Read the model definition and answer for the solid it produces. Units are mm, in the model's axes. A direction names the side the tool comes from. Coordinates: 2 decimals unless noted, no trailing zeros. Order: outer loops, then holes, each group sorted by start corner. A loop starts at its lowest first (then second) coordinate and runs counter-clockwise, first axis right, second up. Notation, with made-up numbers: (43, 20) -> (94, 20) arc R37 ccw to (94, 57) -> close; hole circle Ø2 at (-1.75, -36.75). An arc over 180 degrees is marked (long way). Answer as a JSON object with one key per item and string values. Group by question number.
1) A tool of negligible diameter and unlimited length cuts with its end or side. For faces 1 (the flat face through (-6, -19.05, 19)), 2 (the flat face through (0, -24, 22)), 3 (the flat face through (-6, -28, 25.4)), from which of +Z, -Z, +X, -X, +Y, -Y can it reach the whole face along a straight path? Write none if from no direction.
2) Section B-B on y = -25.5 is taken. Determine the outline of the cut face in (x, z), and give its area (3 significant figures).
3) Consider L1, parallel to Y at x = -6.5, z = 23; L2, parallel to X at y = -3, z = 9.5; L3, parallel to Z at x = -1, y = -9.5. Determine where each line is inside the solid, lowest interval first.
4) Given pin 1 (8 mm diameter, centred on x = -8, z = 18.5, fed in from +Y); pin 2 (6 mm diameter, centred on x = 3.5, y = -4.5, fed in from +Z); pin 3 (12 mm diameter, centred on x = 9.5, y = -27.5, fed in from +Z), each flat-ended and moving along its own axis, determine where each tip first touches the part or whether it passes through.
5) Section A-A on x = -6 is taken. Determine the outline of the cut face in (y, z), and give its area (3 significant figures).
from build123d import *

# Parameters (mm, degrees)
F0_W     = 38.1
F0_H     = 25.4
F1_DEPTH = 12.7
F2_SIZE2 = 25.39999
F2_SIZE  = 38.09999
F4_DEPTH = 12.7


# Not quite as in the source:
# - a fillet or chamfer is up to 0.001 mm smaller than in the source, because OpenCascade refuses the exact size


with BuildPart() as f1:
    # F0 (on Right) → F1 (new body)
    with BuildSketch(Plane.YZ):
        with Locations((-19.05, 12.7)):
            Rectangle(F0_W, F0_H)
    extrude(amount=F1_DEPTH)

    # F2 (size 38.1 and 25.4 in the source; OpenCascade refuses exactly that, so slightly less here)
    f2_edges = [f1.edges().sort_by_distance(p)[0] for p in [
        (6.35, 0, 25.4),
    ]]
    f2_side = f1.faces().sort_by_distance((6.35, -19.05, 25.4))[0]
    chamfer(f2_edges, length=F2_SIZE, length2=F2_SIZE2, reference=f2_side)

    # F3 (on Right) → F4 (join)
    with BuildSketch(Plane.YZ):
        Polygon((-38.1, 0), (0, 0), (0, 12.7), (-19.05, 12.7), (-19.05, 25.4), (-38.1, 25.4), align=None)
    extrude(amount=-F4_DEPTH)


solid = f1.part
Worked answers:
{
 "1": {"face 1": "+Z, +X, -X, +Y", "face 2": "+Z, +X, +Y", "face 3": "+Z, +X, -X, +Y, -Y"},
 "2": {"outline": "(-12.7, 0) -> (12.7, 0) -> (12.7, 17) -> (0, 17) -> (0, 25.4) -> (-12.7, 25.4) -> close", "area": "538 mm²"},
 "3": {"L1": "y = -38.1 to -19.05", "L2": "x = -12.7 to 0", "L3": "z = 0 to 12.7"},
 "4": {"pin 1": "stops at y = -19.05", "pin 2": "stops at z = 5", "pin 3": "stops at z = 22.33"},
 "5": {"outline": "(-38.1, 0) -> (0, 0) -> (0, 12.7) -> (-19.05, 12.7) -> (-19.05, 25.4) -> (-38.1, 25.4) -> close", "area": "726 mm²"}
}
